```python
from build123d import *

# Parameters (mm, degrees)
SKETCH1_R                 = 1.651
BOSS_EXTRUDE2_DEPTH       = 5.3975
SKETCH2_R                 = 1.143
CUT_EXTRUDE1_DEPTH        = 6.3975
SKETCH3_R                 = 12.1285
CUT_EXTRUDE2_DEPTH        = 6.3975
SKETCH4_W                 = 28.562713242
SKETCH4_H                 = 11.677503754
BOSS_EXTRUDE3_DEPTH       = 5.3975
SKETCH5_W                 = 216.7214489
SKETCH5_H                 = 130.569220634
CUT_EXTRUDE4_DEPTH        = 6.3975
SKETCH6_R                 = 38.1
CUT_EXTRUDE5_DEPTH        = 60.96
FILLET1_R                 = 6.35
FILLET2_R                 = 6.35
SKETCH102_W               = 11.43
SKETCH102_H               = 10.16
CUT_EXTRUDE101_DEPTH      = 6.3975001
SKETCH158_R               = 1.651
CUT_EXTRUDE157_DEPTH      = 97.79
SKETCH212_R               = 3.175
CUT_EXTRUDE211_DEPTH      = 103.378
CUT_EXTRUDE211_DEPTH_BACK = 48.768
CUT_EXTRUDE104_DEPTH      = 10
FILLET3_R                 = 2.54
SKETCH225_R               = 12.1285
BOSS_EXTRUDE4_DEPTH       = 5.3975
CUT_EXTRUDE224_DEPTH      = 6.3975001


with BuildPart() as part:
    # Sketch1 → Boss-Extrude2 (new body)
    with BuildSketch(Plane.XY):
        with BuildLine():
            Line((-64.964441474, 37.338), (-54.550441474, 37.338))
            Line((-54.550441474, 37.338), (-54.550441474, -37.338))
            Line((-54.550441474, -37.338), (-64.964441474, -37.338))
            ThreePointArc((-64.964441474, -37.338), (0, -74.93), (64.964441474, -37.338))
            Line((64.964441474, -37.338), (54.550441474, -37.338))
            Line((54.550441474, -37.338), (54.550441474, 37.338))
            Line((54.550441474, 37.338), (64.964441474, 37.338))
            ThreePointArc((64.964441474, 37.338), (0, 74.93), (-64.964441474, 37.338))
        make_face()
        with Locations((-46.482, 11.049)):
            Circle(SKETCH1_R, mode=Mode.SUBTRACT)
        with Locations((-21.083270032, 10.795)):
            Circle(SKETCH1_R, mode=Mode.SUBTRACT)
        with Locations((-21.083270032, -10.795)):
            Circle(SKETCH1_R, mode=Mode.SUBTRACT)
        with Locations((-46.482, -11.049)):
            Circle(SKETCH1_R, mode=Mode.SUBTRACT)
        with Locations((46.482, -11.049)):
            Circle(SKETCH1_R, mode=Mode.SUBTRACT)
        with Locations((21.083270032, -10.795)):
            Circle(SKETCH1_R, mode=Mode.SUBTRACT)
        with Locations((21.083270032, 10.795)):
            Circle(SKETCH1_R, mode=Mode.SUBTRACT)
        with Locations((46.482, 11.049)):
            Circle(SKETCH1_R, mode=Mode.SUBTRACT)
    extrude(amount=BOSS_EXTRUDE2_DEPTH)

    # Sketch2 → Cut-Extrude1 (cut, through all)
    with BuildSketch(Plane.XY.offset(5.3975)):
        with Locations((-6.731, 62.23)):
            Circle(SKETCH2_R)
        with Locations((6.731, 62.23)):
            Circle(SKETCH2_R)
    extrude(amount=-CUT_EXTRUDE1_DEPTH, mode=Mode.SUBTRACT)

    # Sketch3 → Cut-Extrude2 (cut, through all)
    with BuildSketch(Plane(origin=(0, 0, 0), x_dir=(-1, 0, 0), z_dir=(0, 0, -1))):
        with Locations((-43.105229381, -43.105229381)):
            Circle(SKETCH3_R)
        with Locations((14.224, -34.29)):
            Circle(SKETCH3_R)
        with Locations((14.224, 34.29)):
            Circle(SKETCH3_R)
        with Locations((-43.105229381, 43.105229381)):
            Circle(SKETCH3_R)
        with Locations((43.105229381, 43.105229381)):
            Circle(SKETCH3_R)
        with Locations((-14.224, 34.29)):
            Circle(SKETCH3_R)
        with Locations((-14.224, -34.29)):
            Circle(SKETCH3_R)
        with Locations((43.105229381, -43.105229381)):
            Circle(SKETCH3_R)
    extrude(amount=-CUT_EXTRUDE2_DEPTH, mode=Mode.SUBTRACT)

    # Sketch4 → Boss-Extrude3 (add)
    with BuildSketch(Plane(origin=(0, 0, 0), x_dir=(-1, 0, 0), z_dir=(0, 0, -1))):
        with Locations((-1.488809975, 62.152540216)):
            Rectangle(SKETCH4_W, SKETCH4_H)
    extrude(amount=-BOSS_EXTRUDE3_DEPTH)

    # Sketch5 → Cut-Extrude4 (cut, through all)
    with BuildSketch(Plane(origin=(0, 0, 0), x_dir=(-1, 0, 0), z_dir=(0, 0, -1))):
        with Locations((23.316688373, 48.139610317)):
            Rectangle(SKETCH5_W, SKETCH5_H)
    extrude(amount=-CUT_EXTRUDE4_DEPTH, mode=Mode.SUBTRACT)

    # Sketch6 → Cut-Extrude5 (cut)
    with BuildSketch(Plane(origin=(0, 0, 0), x_dir=(-1, 0, 0), z_dir=(0, 0, -1))):
        with Locations((0, -86.312058398)):
            Circle(SKETCH6_R)
    extrude(amount=-CUT_EXTRUDE5_DEPTH, mode=Mode.SUBTRACT)

    # Fillet1
    fillet1_edges = [part.edges().sort_by_distance(p)[0] for p in [
        (-33.000960548, -67.271401821, 2.69875),
    ]]
    fillet(fillet1_edges, radius=FILLET1_R)

    # Fillet2
    fillet2_edges = [part.edges().sort_by_distance(p)[0] for p in [
        (33.000960548, -67.271401821, 2.69875),
    ]]
    fillet(fillet2_edges, radius=FILLET2_R)

    # Sketch102 → Cut-Extrude101 (cut, through all)
    with BuildSketch(Plane(origin=(0, 0, 0), x_dir=(-1, 0, 0), z_dir=(0, 0, -1))):
        with Locations((-33.595441474, -22.225)):
            Rectangle(SKETCH102_W, SKETCH102_H)
        with Locations((33.595441474, -22.225)):
            Rectangle(SKETCH102_W, SKETCH102_H)
    extrude(amount=-CUT_EXTRUDE101_DEPTH, mode=Mode.SUBTRACT)

    # Sketch158 → Cut-Extrude157 (cut)
    with BuildSketch(Plane(origin=(30.092005081, 4.08352975, -24.638), x_dir=(-1, 0, 0), z_dir=(0, 0, -1))):
        with Locations((4.154396091, -49.728759131)):
            Circle(SKETCH158_R)
        with Locations((56.02961407, -49.728759131)):
            Circle(SKETCH158_R)
    extrude(amount=-CUT_EXTRUDE157_DEPTH, mode=Mode.SUBTRACT)

    # Sketch212 → Cut-Extrude211 (cut, two sides)
    with BuildSketch(Plane(origin=(30.092005081, 4.08352975, 11.4935), x_dir=(-1, 0, 0), z_dir=(0, 0, -1))) as cut_extrude211_sk:
        with Locations((77.082005081, -29.48352975)):
            Circle(SKETCH212_R)
        with Locations((30.092005081, -29.48352975)):
            Circle(SKETCH212_R)
        with Locations((-16.897994919, -29.48352975)):
            Circle(SKETCH212_R)
    extrude(amount=CUT_EXTRUDE211_DEPTH, mode=Mode.SUBTRACT)
    extrude(cut_extrude211_sk.sketch, amount=-CUT_EXTRUDE211_DEPTH_BACK, mode=Mode.SUBTRACT)

    # Sketch105 → Cut-Extrude104 (cut)
    with BuildSketch(Plane(origin=(0, 0, 0), x_dir=(-1, 0, 0), z_dir=(0, 0, -1))):
        with BuildLine():
            Line((-12.7, -20.32), (-8.89, -20.32))
            ThreePointArc((-8.89, -20.32), (-5.715, -23.495), (-2.54, -20.32))
            Line((-2.54, -20.32), (2.54, -20.32))
            ThreePointArc((2.54, -20.32), (5.715, -23.495), (8.89, -20.32))
            Line((8.89, -20.32), (12.7, -20.32))
            ThreePointArc((12.7, -20.32), (18.415, -14.605), (12.7, -8.89))
            Line((12.7, -8.89), (-12.7, -8.89))
            ThreePointArc((-12.7, -8.89), (-18.415, -14.605), (-12.7, -20.32))
        make_face()
    extrude(amount=-CUT_EXTRUDE104_DEPTH, mode=Mode.SUBTRACT)

    # Fillet3
    fillet3_edges = [part.edges().sort_by_distance(p)[0] for p in [
        (39.310441474, -17.145, 2.69875),
        (27.880441474, -17.145, 2.69875),
        (-27.880441474, -17.145, 2.69875),
        (-39.310441474, -17.145, 2.69875),
        (17.81953367, -17.145, 2.69875),
        (-17.81953367, -17.145, 2.69875),
        (-8.89, -20.32, 2.69875),
        (-2.54, -20.32, 2.69875),
        (2.54, -20.32, 2.69875),
        (8.89, -20.32, 2.69875),
    ]]
    fillet(fillet3_edges, radius=FILLET3_R)

    # Sketch225 → Boss-Extrude4 (add)
    with BuildSketch(Plane(origin=(0, 0, 0), x_dir=(-1, 0, 0), z_dir=(0, 0, -1))):
        with Locations((-14.224, -34.29)):
            Circle(SKETCH225_R)
        with Locations((14.224, -34.29)):
            Circle(SKETCH225_R)
    extrude(amount=-BOSS_EXTRUDE4_DEPTH)

    # Sketch226 → Cut-Extrude224 (cut, through all)
    with BuildSketch(Plane(origin=(0, 0, 0), x_dir=(-1, 0, 0), z_dir=(0, 0, -1))):
        Polygon((4.445, -37.7228538), (4.445, -40.5091462), (6.858, -41.902292399), (9.271, -40.5091462), (9.271, -37.7228538), (6.858, -36.329707601), align=None)
        Polygon((-4.445, -37.7228538), (-6.858, -36.329707601), (-9.271, -37.7228538), (-9.271, -40.5091462), (-6.858, -41.902292399), (-4.445, -40.5091462), align=None)
    extrude(amount=-CUT_EXTRUDE224_DEPTH, mode=Mode.SUBTRACT)


solid = part.part
```
The listing builds one solid part. Answer for the finished solid, in the listing's coordinates (mm). A direction names the side the tool comes from. Coordinates: 2 decimals unless noted, no trailing zeros. Write each loop counter-clockwise with the first axis right and the second up, starting at its lowest first coordinate (ties: lowest second). Pieces come first, ordered by that corner, then holes. Notation, with made-up numbers: M 10.25,67.25 L 47.25,67.25 A12 cw 47.25,71.25 Z; hole C 60,0.25 d8. An arc over 180 degrees is marked long. Use a Markdown table: item, result. Add a question column.
1. Section C-C (y = -35) is taken. Give the vertices of the cut face in (x, z).
2. Which of the six approach directions +Z, -Z, +X, -X, +Y, -Y give full straight-line access (tool end or side, diameter ignored) to faces 1 (the flat face through (5.63, -37.04, 2.66)), 2 (the flat face through (-39.31, -24, 3)), 3 (the cylindrical face through (53.178, -52.788, 2.661)), 4 (the flat face through (60, -37.338, 3))?
3. Given P1, Ø3, axis at x = -18, y = -54, coming from the -Z side; P2, Ø1.5, axis at x = 36.5, z = 2.5, coming from the +Y side (3 decimals); P3, Ø1, axis at y = -50.5, z = 4, coming from the -X side; P4, Ø2.5, axis at x = -61, z = 2, coming from the +Y side, each flat-ended and moving along its own axis, determine where each tip first touches the part or whether it passes through.
4. Section B-B (x = -46.99) is taken. Give the vertices of the cut face in (y, z) (1 decimal), plus the area to 3 significant figures.
5. Section A-A (y = -25.4) is taken. Give the vertices of the cut face in (x, z) (1 decimal), plus the area to 3 significant figures.
6. For a pull along X with two mould halves and no side action, classify faces 5 (the flat face through (-4.445, -39, 3)), 6 (the flat face through (-9.271, -39, 3)), 7 (the flat face through (1, -41, 0)), 8 (the flat face through (-54.55, -27, 3)) as +X half, -X half, draft (parallel to the pull), parting line (faces both ways), or undercut.
7. Straight lines are drawn through the part: line 1 along X through (y, z) = (-25.4, 1.3) (3 decimals); line 2 along X through (y, z) = (-47.5, 3.9); line 3 along Y through (x, z) = (-49, 3.95) (3 decimals). For each, find the intervals that lie inside material, in ascending order. Write a range as [from, to].
8. Section D-D (y = -50) is taken. Give the vertices of the cut face in (x, z).
Data:
| question | item | result |
|---|---|---|
| 1 | outline | M -54.55,0 L -52.13,0 L -52.13,5.4 L -54.55,5.4 Z; M -34.08,0 L 34.08,0 L 34.08,5.4 L -34.08,5.4 Z; M 52.13,0 L 54.55,0 L 54.55,5.4 L 52.13,5.4 Z |
| 2 | face 1 | +Z, -Z |
| 2 | face 2 | +Z, -Z, +Y |
| 2 | face 3 | +Z, -Z, +X, -Y |
| 2 | face 4 | +Z, -Z, +X, +Y |
| 3 | P1 | stops at z = 0 |
| 3 | P2 | stops at y = -27.305 |
| 3 | P3 | stops at x = -55.81 |
| 3 | P4 | stops at y = -37.34 |
| 4 | outline | M -58.4,0 L -54.6,0 L -54.6,5.4 L -58.4,5.4 Z; M -31.6,0 L -28.6,0 L -28.6,5.4 L -31.6,5.4 Z; M -22.2,0 L -17.1,0 L -17.1,5.4 L -22.2,5.4 Z |
| 4 | area | 64.2 mm2 |
| 5 | outline | M -54.6,0 L -50.2,0 L -50.2,5.4 L -54.6,5.4 Z; M -43.8,0 L -39.3,0 L -39.3,5.4 L -43.8,5.4 Z; M -27.9,0 L -3.2,0 L -3.2,5.4 L -27.9,5.4 Z; M 3.2,0 L 27.9,0 L 27.9,5.4 L 3.2,5.4 Z; M 39.3,0 L 43.8,0 L 43.8,5.4 L 39.3,5.4 Z; M 50.2,0 L 54.6,0 L 54.6,5.4 L 50.2,5.4 Z |
| 5 | area | 363 mm2 |
| 6 | face 5 | undercut |
| 6 | face 6 | undercut |
| 6 | face 7 | draft |
| 6 | face 8 | -X half |
| 7 | line 1 | x = [-54.55, -50.165], [-43.815, -39.31], [-27.88, -3.175], [3.175, 27.88], [39.31, 43.815], [50.165, 54.55] |
| 7 | line 2 | x = [-57.95, -54.41], [-31.8, 31.8], [54.41, 57.95] |
| 7 | line 3 | y = [-56.688, -53.705], [-32.506, -27.858], [-22.942, -17.145] |
| 8 | outline | M -55.81,0 L -53.08,0 L -53.08,5.4 L -55.81,5.4 Z; M -33.13,0 L -11.53,0 L -11.53,5.4 L -33.13,5.4 Z; M 11.53,0 L 33.13,0 L 33.13,5.4 L 11.53,5.4 Z; M 53.08,0 L 55.81,0 L 55.81,5.4 L 53.08,5.4 Z |
